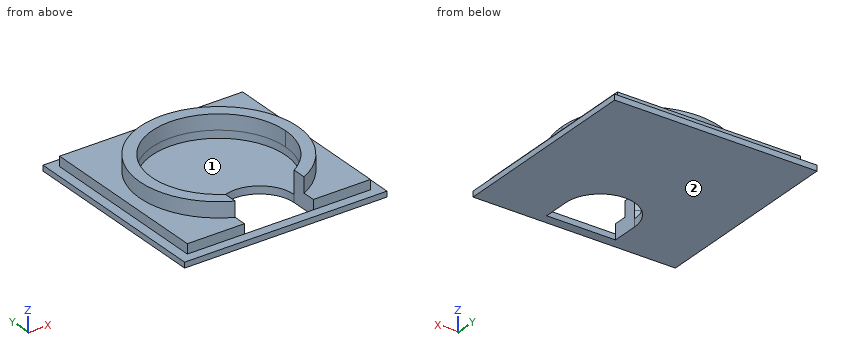
from build123d import *
from build123d.topology import SkipClean

# Parameters (mm, degrees)
SKETCH16_W           = 60.3
SKETCH16_H           = 58.8
SKETCH16_R           = 22
BOSS_EXTRUDE2_DEPTH  = 5
SKETCH22_W           = 60.3
SKETCH22_H           = 2.5
BOSS_EXTRUDE7_DEPTH  = 50
BOSS_EXTRUDE8_START  = 5
BOSS_EXTRUDE8_DEPTH  = 5
SKETCH27_W           = 66.65
SKETCH27_H           = 65.15
BOSS_EXTRUDE10_DEPTH = 1.825
CUT_EXTRUDE3_DEPTH   = 26.375


with BuildPart() as part:
    # Sketch16 → Boss-Extrude2 (new body)
    with BuildSketch(Plane.XY):
        with Locations((0, 1.75)):
            Rectangle(SKETCH16_W, SKETCH16_H)
        Circle(SKETCH16_R, mode=Mode.SUBTRACT)
    extrude(amount=-BOSS_EXTRUDE2_DEPTH)

    # Sketch22 → Boss-Extrude7 (add)
    with BuildSketch(Plane(origin=(0, 31.15, 0), x_dir=(1, 0, 0), z_dir=(0, 1, 0))):
        with Locations((0, 3.75)):
            Rectangle(SKETCH22_W, SKETCH22_H)
    extrude(amount=-BOSS_EXTRUDE7_DEPTH)

    # Sketch23 → Boss-Extrude8 (add)
    with SkipClean():  # the faces are left unmerged after this step: merging them gives an invalid solid
        with BuildSketch(Plane.XY.offset(BOSS_EXTRUDE8_START)):
            with BuildLine():
                ThreePointArc((26, 0), (-13.803371437, 22.033314253), (-11.343610536, -23.394924663))
                Line((-11.343610536, -23.394924663), (-11.343610536, -18.85))
                ThreePointArc((-11.343610536, -18.85), (-10.826831674, 19.151493829), (22, 0))
                Line((22, 0), (22, -13.856406461))
                ThreePointArc((22, -13.856406461), (24.979991994, -7.211102551), (26, 0))
            make_face()
            with BuildLine():
                Line((11.343610536, -18.85), (11.343610536, -23.394924663))
                ThreePointArc((11.343610536, -23.394924663), (17.340557179, -19.372792177), (22, -13.856406461))
                Line((22, -13.856406461), (22, 0))
                ThreePointArc((22, 0), (19.151493829, -10.826831674), (11.343610536, -18.85))
            make_face()
        extrude(amount=-BOSS_EXTRUDE8_DEPTH)

    # Sketch27 → Boss-Extrude10 (add)
    with SkipClean():  # the faces are left unmerged after this step: merging them gives an invalid solid
        with BuildSketch(Plane.XY.offset(-3.175)):
            with Locations((0, 1.75)):
                Rectangle(SKETCH27_W, SKETCH27_H)
        extrude(amount=-BOSS_EXTRUDE10_DEPTH)

    # Sketch24 → Cut-Extrude3 (cut, symmetric)
    with SkipClean():  # the faces are left unmerged after this step: merging them gives an invalid solid
        with BuildSketch(Plane.XY.offset(-2.5)):
            with BuildLine():
                Line((-11.343610536, -18.85), (-11.343610536, -27.65))
                Line((-11.343610536, -27.65), (11.343610536, -27.65))
                Line((11.343610536, -27.65), (11.343610536, -18.85))
                ThreePointArc((11.343610536, -18.85), (0, -7.506389464), (-11.343610536, -18.85))
            make_face()
        extrude(amount=CUT_EXTRUDE3_DEPTH, both=True, mode=Mode.SUBTRACT)


solid = part.part
Model file for the job. Use its own axes, mm. Face numbers are marked on the shaded views. Give positions to 0.01 mm unless a question says otherwise; leave off trailing zeros. Loops run counter-clockwise (first coordinate to the right, second up) from the corner with the lowest first, then second, coordinate; pieces in that order, holes last.
1) Saw through at C-C (x = -24). Write the cut outline in (y, z) (3 decimals).
2) Saw through at D-D (y = 19.5). Write the cut outline in (x, z) (3 decimals), plus the area to 3 significant figures.
3) Saw through at B-B (z = 1). Write the cut outline in (x, y), plus the area to 3 significant figures.
4) Pull direction Y, two halves, no side cores. Call the marked faces 1 and 2: +Y half, -Y half, draft (parallel to the pull), parting line (faces both ways), or undercut.
5) Saw through at A-A (x = 0). Write the cut outline in (y, z) (3 decimals).
6) Flat gauge pins, fed straight in: pin 1 Ø3.5 at (x, z) = (-18.5, -1) entering from -Y; pin 2 Ø1.6 at (y, z) = (15, -1.5) entering from -X; pin 3 Ø10 at (x, y) = (-26.5, -20) entering from +Z. Where does each tip first touch, or does it go through?
7) Wall check: line 1 (Z direction, x = 19.5, y = -18); line 2 (X direction, y = 0, z = -0.7); line 3 (Z direction, x = -19.5, y = 4). Give the ranges that are in metal, low to high.
Answer block:
1. outline: (-30.825, -5) - (34.325, -5) - (34.325, -3.175) - (31.15, -3.175) - (31.15, 0) - (10, 0) - (10, 5) - (-10, 5) - (-10, 0) - (-27.65, 0) - (-27.65, -3.175) - (-30.825, -3.175) - close
2. outline: (-33.325, -5) - (33.325, -5) - (33.325, -3.175) - (30.15, -3.175) - (30.15, 0) - (17.197, 0) - (17.197, 5) - (10.186, 5) - (10.186, -2.5) - (-10.186, -2.5) - (-10.186, 5) - (-17.197, 5) - (-17.197, 0) - (-30.15, 0) - (-30.15, -3.175) - (-33.325, -3.175) - close
2. area: 332 mm2
3. outline: (-11.34, -23.39) - (-11.34, -18.85) arc R22 cw (long way) to (11.34, -18.85) - (11.34, -23.39) arc R26 ccw (long way) to start
3. area: 509 mm2
4. face 1: undercut
4. face 2: draft
5. outline: (-30.825, -5) - (-27.65, -5) - (-27.65, -3.175) - (-30.825, -3.175) - close; (-7.506, -5) - (34.325, -5) - (34.325, -3.175) - (31.15, -3.175) - (31.15, 0) - (26, 0) - (26, 5) - (22, 5) - (22, -2.5) - (-7.506, -2.5) - close
6. pin 1: stops at y = -27.65
6. pin 2: stops at x = -30.15
6. pin 3: stops at z = 0
7. line 1: z = -5 to 0
7. line 2: x = -30.15 to -22, 22 to 30.15
7. line 3: z = -5 to -2.5
